Verification items for this drawing (mm, ordinates from the low corner). Round coordinates to 2 decimals unless told otherwise and drop trailing zeros. Write each loop counter-clockwise with the first axis right and the second up, starting at its lowest first coordinate (ties: lowest second). Pieces come first, ordered by that corner, then holes.
Item 1: Draft check along Y on the marked faces 1, 2 and 3. Enter one of: pulls with the +Y half, pulls with the -Y half, needs draft (parallel to the pull), parting line crosses it, or undercut.
Item 2: Depth check by flat-ended pin: P1, Ø2.5, axis at x = 6, y = 1.5, coming from the +Z side; P2, Ø1, axis at x = 8, y = 7, coming from the -Z side; P3, Ø1, axis at x = 2.5, y = 6.5, coming from the +Z side. Enter the tip coordinate at first touch or a pass-through.
Item 3: Cross-section at A-A (x = 6). Enter the section's corners in (y, z).
Item 4: Scan lines: probe 1 along Z at (x, y) = (7, 1.75); probe 2 along Z at (x, y) = (6.75, 7.5); probe 3 along X at (y, z) = (0.5, 4). Record each from-to range of solid material in increasing order.
Item 5: Cross-section at B-B (z = 6). Enter the section's corners in (x, y), then the cut area to 3 significant figures.
Item 6: Cross-section at D-D (y = 3.75). Enter the section's corners in (x, z), then the cut area to 3 significant figures.
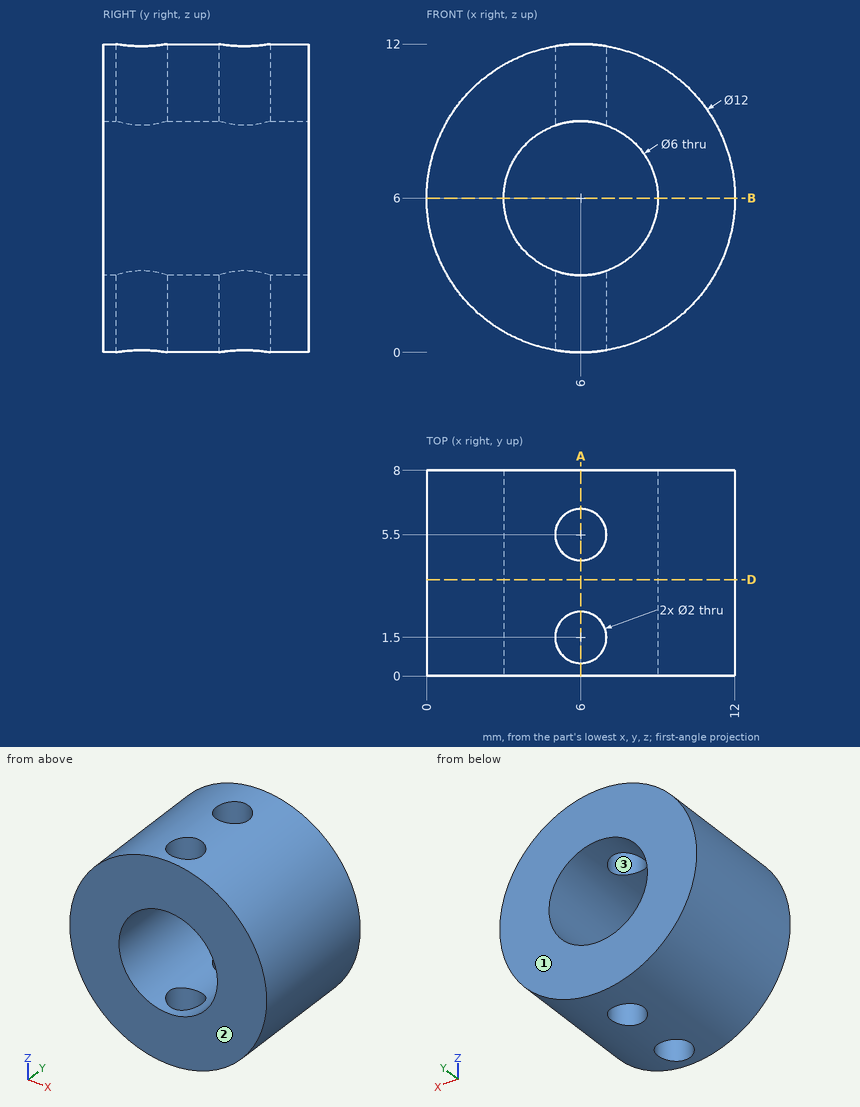
Resolved:
1. face 1: pulls with the +Y half
1. face 2: pulls with the -Y half
1. face 3: undercut
2. P1: stops at z = 12
2. P2: stops at z = 0.19
2. P3: stops at z = 11.2
3. outline: (0, 0) - (0.5, 0) - (0.5, 3) - (0, 3) - close; (0, 9) - (0.5, 9) - (0.5, 12) - (0, 12) - close; (2.5, 0) - (4.5, 0) - (4.5, 3) - (2.5, 3) - close; (2.5, 9) - (4.5, 9) - (4.5, 12) - (2.5, 12) - close; (6.5, 0) - (8, 0) - (8, 3) - (6.5, 3) - close; (6.5, 9) - (8, 9) - (8, 12) - (6.5, 12) - close
4. probe 1: z = 0.08 to 3.17, 8.83 to 11.92
4. probe 2: z = 0.05 to 3.1, 8.9 to 11.95
4. probe 3: x = 0.34 to 3.76, 8.24 to 11.66
5. outline: (0, 0) - (3, 0) - (3, 8) - (0, 8) - close; (9, 0) - (12, 0) - (12, 8) - (9, 8) - close
5. area: 48.0 mm2
6. outline: circle Ø12 at (6, 6); hole circle Ø6 at (6, 6)
6. area: 84.8 mm2
